Can you work these out from the model? Positions are in its coordinate system, mm. Face numbers are marked on the shaded views. Give positions to 0.01 mm unless a question says otherwise; leave off trailing zeros. Write each loop counter-clockwise with the first axis right and the second up, starting at its lowest first coordinate (ties: lowest second). Pieces come first, ordered by that corner, then holes.
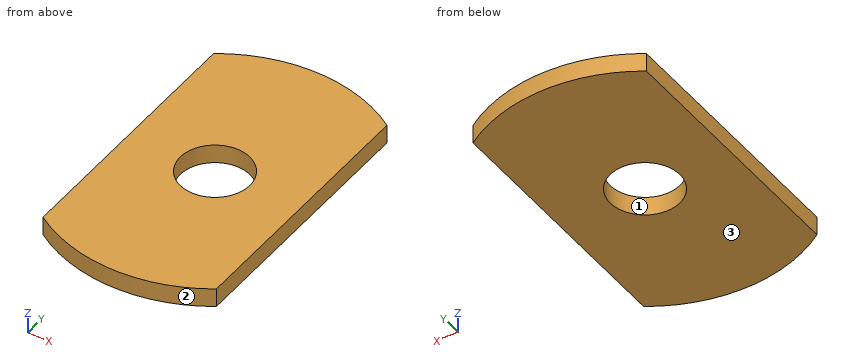
```python
from build123d import *

# Parameters (mm, degrees)
SKETCH1_R      = 1.5875
EXTRUDE1_DEPTH = 0.8636


with BuildPart() as part:
    # Sketch1 → Extrude1 (new body)
    with BuildSketch(Plane.XY):
        with BuildLine():
            Line((-3.9624, 5.936485913), (-3.9624, -5.936485913))
            ThreePointArc((-3.9624, -5.936485913), (0, -7.1374), (3.9624, -5.936485913))
            Line((3.9624, -5.936485913), (3.9624, 5.936485913))
            ThreePointArc((3.9624, 5.936485913), (0, 7.1374), (-3.9624, 5.936485913))
        make_face()
        Circle(SKETCH1_R, mode=Mode.SUBTRACT)
    extrude(amount=-EXTRUDE1_DEPTH)


solid = part.part
```
1) Suppose I cut it at A-A on y = 0. Write out the boundary of the cut face in (x, z), plus the area to 3 significant figures.
Values follow:
outline: (-3.96, -0.86) - (-1.59, -0.86) - (-1.59, 0) - (-3.96, 0) - close; (1.59, -0.86) - (3.96, -0.86) - (3.96, 0) - (1.59, 0) - close
area: 4.10 mm2
2) Suppose I cut it at C-C on z = -0.35. Write out the boundary of the cut face in (x, y) (1 decimal), plus the area to 3 significant figures.
Values follow:
outline: (-4, -5.9) arc R7.1 ccw to (4, -5.9) - (4, 5.9) arc R7.1 ccw to (-4, 5.9) - close; hole circle Ø3.2 at (0, 0)
area: 99.1 mm2
3) If we mould it in two halves opening along Y, with no side actions, what happens to the marked faces 1, 2 and 3? For each: +Y half, -Y half, draft (parallel to the pull), parting line (faces both ways), or undercut.
Values follow:
face 1: undercut
face 2: -Y half
face 3: draft
4) For pin 1 Ø3 at (x, y) = (0, 0) entering from -Z, with a flat end and sliding along its axis, tell me the tip position at first contact or that it passes through.
Values follow:
pin 1: passes through
5) Please list where these lines run through material, in increasing order: L1, parallel to Y at x = 0.5, z = -0.45; L2, parallel to Y at x = 0.75, z = -0.25; L3, parallel to Y at x = 2, z = -0.15.
Values follow:
L1: y = -7.12 to -1.51, 1.51 to 7.12
L2: y = -7.1 to -1.4, 1.4 to 7.1
L3: y = -6.85 to 6.85
6) Suppose I cut it at B-B on x = 0. Write out the boundary of the cut face in (y, z), plus the area to 3 significant figures.
Values follow:
outline: (-7.14, -0.86) - (-1.59, -0.86) - (-1.59, 0) - (-7.14, 0) - close; (1.59, -0.86) - (7.14, -0.86) - (7.14, 0) - (1.59, 0) - close
area: 9.59 mm2
7) Suppose I cut it at D-D on x = -2. Write out the boundary of the cut face in (y, z).
Values follow:
outline: (-6.85, -0.86) - (6.85, -0.86) - (6.85, 0) - (-6.85, 0) - close
